Job drawing, mm, ordinate dimensions from the low corner. One solid piece. Give positions to 0.01 mm unless a question says otherwise; leave off trailing zeros. Write each loop counter-clockwise with the first axis right and the second up, starting at its lowest first coordinate (ties: lowest second). Pieces come first, ordered by that corner, then holes. Notation, with made-up numbers: (66.25, 33.5) - (97.25, 33.5) arc R11 ccw to (97.25, 38.5) - close; hole circle Ø11 at (77.5, 17). An arc over 180 degrees is marked (long way). Put each result on its own line as item: value. Start each with the question number.
1. Cut at B-B on x = 33. List the corners of the cut face in (y, z).
2. Mould opens along X. For the marked faces 1, 2, 3 and 4 say: +X half, -X half, draft (parallel to the pull), parting line (faces both ways), or undercut.
3. Cut at A-A on z = 16.35. List the corners of the cut face in (x, y), and give its area (3 significant figures).
4. Cut at C-C on y = 3. List the corners of the cut face in (x, z).
5. Wall check: line 1 (Z direction, x = 33, y = 8.75); line 2 (Z direction, x = 35, y = 14.5) (1 decimal); line 3 (X direction, y = 13.75, z = 14) (1 decimal). Give the ranges that are in metal, low to high.
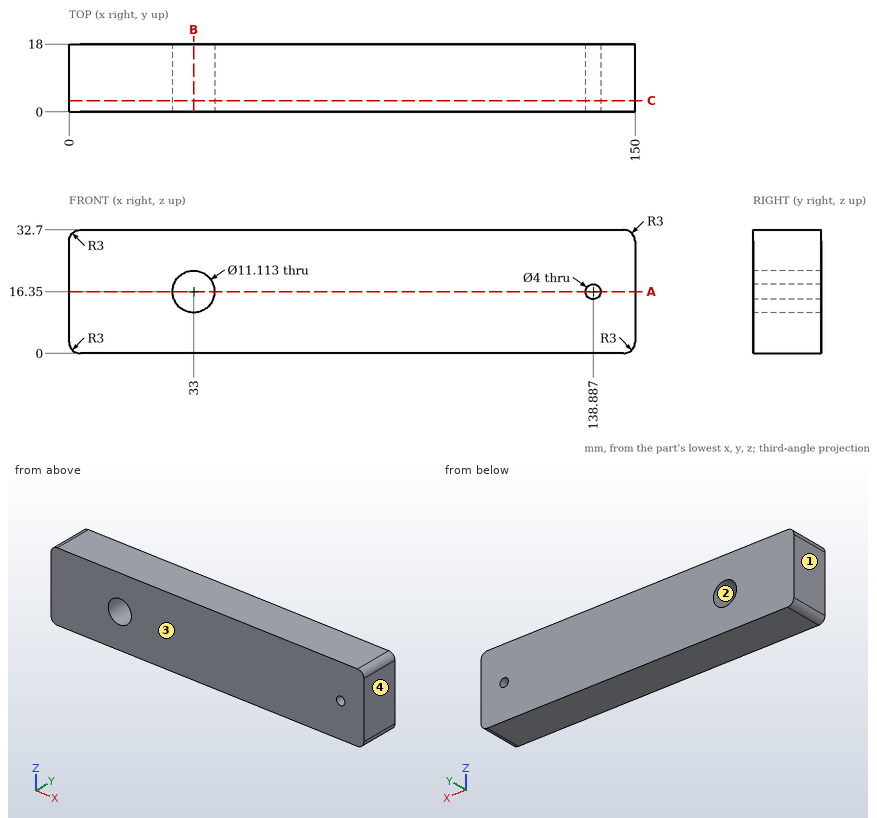
Report:
1. outline: (0, 0) - (18, 0) - (18, 10.79) - (0, 10.79) - close; (0, 21.91) - (18, 21.91) - (18, 32.7) - (0, 32.7) - close
2. face 1: -X half
2. face 2: undercut
2. face 3: draft
2. face 4: +X half
3. outline: (0, 0) - (27.44, 0) - (27.44, 18) - (0, 18) - close; (38.56, 0) - (136.89, 0) - (136.89, 18) - (38.56, 18) - close; (140.89, 0) - (150, 0) - (150, 18) - (140.89, 18) - close
3. area: 2,430 mm²
4. outline: (0, 3) arc R3 ccw to (3, 0) - (147, 0) arc R3 ccw to (150, 3) - (150, 29.7) arc R3 ccw to (147, 32.7) - (3, 32.7) arc R3 ccw to (0, 29.7) - close; hole circle Ø11.11 at (33, 16.35); hole circle Ø4 at (138.89, 16.35)
5. line 1: z = 0 to 10.79, 21.91 to 32.7
5. line 2: z = 0 to 11.2, 21.5 to 32.7
5. line 3: x = 0 to 28, 38 to 150
